Verification items for the finished model (mm, model axes). Round coordinates to 2 decimals unless told otherwise and drop trailing zeros. Order: outer loops, then holes, each group sorted by start corner. A loop starts at its lowest first (then second) coordinate and runs counter-clockwise, first axis right, second up. Notation, with made-up numbers: M -19.75,33.5 L -15.75,33.5 A23 cw -15.75,60.5 Z; hole C 0,-37.75 d2. An arc over 180 degrees is marked long. Use one line per item in the form item = value. Start each with the question number.
Item 1: Thickness scan on probe 1 along X at (y, z) = (12.5, 697); probe 2 along Z at (x, y) = (-23, 8); probe 3 along Z at (x, y) = (16.5, 10.5). Record the ranges inside material, lowest first. Write a range as [from, to].
Item 2: Release check for a two-part mould opening along X. For faces 1 (the flat face through (24.33, 0.27, 687.43)), 2 (the cylindrical face through (-8.142, 0.267, 724.627)), 3 (the flat face through (-1, -19.05, 398)), 4 (the flat face through (-44.45, 0, 398)) record: +X half, -X half, draft (parallel to the pull), parting line (faces both ways), or undercut.
Item 3: Cross-section at B-B on x = 26.5. Enter the section's corners in (y, z).
Item 4: Go/stop test with flat-tipped pins: pin 1 Ø4 at (x, y) = (4, 2.5) entering from -Z; pin 2 Ø10 at (x, y) = (-22.5, -12) entering from -Z. Record where each tip stops, or that it passes through.
Item 5: Cross-section at C-C on z = 710. Enter the section's corners in (x, y).
from build123d import *

# Parameters (mm, degrees)
SKETCH1_W           = 88.9
SKETCH1_H           = 38.1
BOSS_EXTRUDE1_DEPTH = 806.55922
CUT_EXTRUDE1_DEPTH  = 39.1
SKETCH3_R           = 9.525
CUT_EXTRUDE2_DEPTH  = 39.1


with BuildPart() as part:
    # Sketch1 → Boss-Extrude1 (new body)
    with BuildSketch(Plane.XY):
        Rectangle(SKETCH1_W, SKETCH1_H)
    extrude(amount=BOSS_EXTRUDE1_DEPTH)

    # Sketch2 → Cut-Extrude1 (cut, through all)
    with BuildSketch(Plane(origin=(0, 19.05, 0), x_dir=(1, 0, 0), z_dir=(0, 1, 0))):
        Polygon((-44.45, 0), (44.45, 0), (44.45, -51.326438931), align=None)
        Polygon((-44.45, -806.55922), (44.45, -652.579903207), (44.45, -806.55922), align=None)
    extrude(amount=-CUT_EXTRUDE1_DEPTH, mode=Mode.SUBTRACT)

    # Sketch3 → Cut-Extrude2 (cut, through all)
    with BuildSketch(Plane(origin=(0, 19.05, 0), x_dir=(1, 0, 0), z_dir=(0, 1, 0))):
        with Locations((0, -729.569561604)):
            Circle(SKETCH3_R)
    extrude(amount=-CUT_EXTRUDE2_DEPTH, mode=Mode.SUBTRACT)


solid = part.part
Output values:
q1.probe_1 = [-44.45, 18.8]
q1.probe_2 = [12.38, 769.41]
q1.probe_3 = [35.19, 700.99]
q2.face_1 = +X half
q2.face_2 = undercut
q2.face_3 = draft
q2.face_4 = -X half
q3.outline = M -19.05,40.96 L 19.05,40.96 L 19.05,683.67 L -19.05,683.67 Z
q4.pin_1 = 26.82
q4.pin_2 = 9.79
q5.outline = M -44.45,-19.05 L 11.3,-19.05 L 11.3,19.05 L -44.45,19.05 Z
